Source: CAD feature listing. Evaluate the final solid. Frame: model axes, mm. A direction names the side the tool comes from. Give positions to 0.01 mm unless a question says otherwise; leave off trailing zeros. Loops run counter-clockwise (first coordinate to the right, second up) from the corner with the lowest first, then second, coordinate; pieces in that order, holes last. Notation, with made-up numbers: M -37.5,-9.5 L -31.5,-9.5 A15 cw -31.5,18.5 Z; hole C -26.75,33.25 d9. An arc over 180 degrees is marked long. Put each result on its own line as item: value. Start each with the question number.
```python
from build123d import *

# Parameters (mm, degrees)
SKETCH1_R           = 33.02
SKETCH1_R_2         = 22.225
BOSS_EXTRUDE1_DEPTH = 25.4
CAVITY1_DEPTH       = 25.4
CAVITY1_START       = 11.43
CAVITY1_2_DEPTH     = 2.54


# Read off the part's stored shape, not the designer's step: Cavity1
with BuildPart() as part:
    # Sketch1 → Boss-Extrude1 (new body)
    with BuildSketch(Plane(origin=(0, 0, 0), x_dir=(1, 0, 0), z_dir=(0, 1, 0))):
        with Locations(Location((0, 0, 0), (0, 0, 270))):
            Circle(SKETCH1_R)
        with Locations(Location((0, 0, 0), (0, 0, 270))):
            Circle(SKETCH1_R_2, mode=Mode.SUBTRACT)
    extrude(amount=BOSS_EXTRUDE1_DEPTH)

    # Cavity1 outline → Cavity1 (cut)
    with BuildSketch(Plane(origin=(0, 0, 0), x_dir=(1, 0, 0), z_dir=(0, 1, 0))):
        with BuildLine():
            Line((-6.35, -27.94), (6.35, -27.94))
            Line((6.35, -27.94), (2.54, -22.079380086))
            ThreePointArc((2.54, -22.079380086), (0, -22.225), (-2.54, -22.079380086))
            Line((-2.54, -22.079380086), (-6.35, -27.94))
        make_face()
        with BuildLine():
            Line((10.923030829, -19.355568256), (11.285462035, -26.336371175))
            Line((11.285462035, -26.336371175), (21.559977863, -18.871498471))
            Line((21.559977863, -18.871498471), (15.03283716, -16.369619174))
            ThreePointArc((15.03283716, -16.369619174), (13.063527232, -17.9804027), (10.923030829, -19.355568256))
        make_face()
        with BuildLine():
            Line((-11.285462035, -26.336371175), (-10.923030829, -19.355568256))
            ThreePointArc((-10.923030829, -19.355568256), (-13.063527232, -17.9804027), (-15.03283716, -16.369619174))
            Line((-15.03283716, -16.369619174), (-21.559977863, -18.871498471))
            Line((-21.559977863, -18.871498471), (-11.285462035, -26.336371175))
        make_face()
        with BuildLine():
            ThreePointArc((21.783641473, -4.407220121), (21.137231075, -6.8679027), (20.213835141, -9.238587223))
            Line((20.213835141, -9.238587223), (24.610261151, -14.673143701))
            Line((24.610261151, -14.673143701), (28.53477698, -2.594725944))
            Line((28.53477698, -2.594725944), (21.783641473, -4.407220121))
        make_face()
        with BuildLine():
            Line((-24.610261151, -14.673143701), (-20.213835141, -9.238587223))
            ThreePointArc((-20.213835141, -9.238587223), (-21.137231075, -6.8679027), (-21.783641473, -4.407220121))
            Line((-21.783641473, -4.407220121), (-28.53477698, -2.594725944))
            Line((-28.53477698, -2.594725944), (-24.610261151, -14.673143701))
        make_face()
        with BuildLine():
            Line((-28.53477698, 2.594725944), (-21.783641473, 4.407220121))
            ThreePointArc((-21.783641473, 4.407220121), (-21.137231075, 6.8679027), (-20.213835141, 9.238587223))
            Line((-20.213835141, 9.238587223), (-24.610261151, 14.673143701))
            Line((-24.610261151, 14.673143701), (-28.53477698, 2.594725944))
        make_face()
        with BuildLine():
            Line((21.783641473, 4.407220121), (28.53477698, 2.594725944))
            Line((28.53477698, 2.594725944), (24.610261151, 14.673143701))
            Line((24.610261151, 14.673143701), (20.213835141, 9.238587223))
            ThreePointArc((20.213835141, 9.238587223), (21.137231075, 6.8679027), (21.783641473, 4.407220121))
        make_face()
        with BuildLine():
            Line((-21.559977863, 18.871498471), (-15.03283716, 16.369619174))
            ThreePointArc((-15.03283716, 16.369619174), (-13.063527232, 17.9804027), (-10.923030829, 19.355568256))
            Line((-10.923030829, 19.355568256), (-11.285462035, 26.336371175))
            Line((-11.285462035, 26.336371175), (-21.559977863, 18.871498471))
        make_face()
        with BuildLine():
            ThreePointArc((10.923030829, 19.355568256), (13.063527232, 17.9804027), (15.03283716, 16.369619174))
            Line((15.03283716, 16.369619174), (21.559977863, 18.871498471))
            Line((21.559977863, 18.871498471), (11.285462035, 26.336371175))
            Line((11.285462035, 26.336371175), (10.923030829, 19.355568256))
        make_face()
        with BuildLine():
            Line((-6.35, 27.94), (-2.54, 22.079380086))
            ThreePointArc((-2.54, 22.079380086), (0, 22.225), (2.54, 22.079380086))
            Line((2.54, 22.079380086), (6.35, 27.94))
            Line((6.35, 27.94), (-6.35, 27.94))
        make_face()
    extrude(amount=CAVITY1_DEPTH, mode=Mode.SUBTRACT)

    # Cavity1 2 outline → Cavity1 2 (cut)
    with BuildSketch(Plane(origin=(0, 0, 0), x_dir=(1, 0, 0), z_dir=(0, 1, 0)).offset(CAVITY1_START)):
        with BuildLine():
            Line((2.54, -22.079380086), (5.935416317, -27.3022789))
            ThreePointArc((5.935416317, -27.3022789), (8.633934823, -26.572519065), (11.246024223, -25.576757793))
            Line((11.246024223, -25.576757793), (10.923030829, -19.355568256))
            ThreePointArc((10.923030829, -19.355568256), (6.8679027, -21.137231075), (2.54, -22.079380086))
        make_face()
        with BuildLine():
            ThreePointArc((-11.246024223, -25.576757793), (-8.633934823, -26.572519065), (-5.935416317, -27.3022789))
            Line((-5.935416317, -27.3022789), (-2.54, -22.079380086))
            ThreePointArc((-2.54, -22.079380086), (-6.8679027, -21.137231075), (-10.923030829, -19.355568256))
            Line((-10.923030829, -19.355568256), (-11.246024223, -25.576757793))
        make_face()
        with BuildLine():
            ThreePointArc((20.213835141, -9.238587223), (17.9804027, -13.063527232), (15.03283716, -16.369619174))
            Line((15.03283716, -16.369619174), (20.84972956, -18.599257438))
            ThreePointArc((20.84972956, -18.599257438), (22.603934823, -16.422719949), (24.131865747, -14.08178453))
            Line((24.131865747, -14.08178453), (20.213835141, -9.238587223))
        make_face()
        with BuildLine():
            Line((-20.84972956, -18.599257438), (-15.03283716, -16.369619174))
            ThreePointArc((-15.03283716, -16.369619174), (-17.9804027, -13.063527232), (-20.213835141, -9.238587223))
            Line((-20.213835141, -9.238587223), (-24.131865747, -14.08178453))
            ThreePointArc((-24.131865747, -14.08178453), (-22.603934823, -16.422719949), (-20.84972956, -18.599257438))
        make_face()
        with BuildLine():
            ThreePointArc((21.783641473, 4.407220121), (22.225, 0), (21.783641473, -4.407220121))
            Line((21.783641473, -4.407220121), (27.800154768, -2.7919518))
            ThreePointArc((27.800154768, -2.7919518), (27.94, 0), (27.800154768, 2.7919518))
            Line((27.800154768, 2.7919518), (21.783641473, 4.407220121))
        make_face()
        with BuildLine():
            Line((-27.800154768, -2.7919518), (-21.783641473, -4.407220121))
            ThreePointArc((-21.783641473, -4.407220121), (-22.225, 0), (-21.783641473, 4.407220121))
            Line((-21.783641473, 4.407220121), (-27.800154768, 2.7919518))
            ThreePointArc((-27.800154768, 2.7919518), (-27.94, 0), (-27.800154768, -2.7919518))
        make_face()
        with BuildLine():
            Line((-24.131865747, 14.08178453), (-20.213835141, 9.238587223))
            ThreePointArc((-20.213835141, 9.238587223), (-17.9804027, 13.063527232), (-15.03283716, 16.369619174))
            Line((-15.03283716, 16.369619174), (-20.84972956, 18.599257438))
            ThreePointArc((-20.84972956, 18.599257438), (-22.603934823, 16.422719949), (-24.131865747, 14.08178453))
        make_face()
        with BuildLine():
            ThreePointArc((15.03283716, 16.369619174), (17.9804027, 13.063527232), (20.213835141, 9.238587223))
            Line((20.213835141, 9.238587223), (24.131865747, 14.08178453))
            ThreePointArc((24.131865747, 14.08178453), (22.603934823, 16.422719949), (20.84972956, 18.599257438))
            Line((20.84972956, 18.599257438), (15.03283716, 16.369619174))
        make_face()
        with BuildLine():
            Line((-11.246024223, 25.576757793), (-10.923030829, 19.355568256))
            ThreePointArc((-10.923030829, 19.355568256), (-6.8679027, 21.137231075), (-2.54, 22.079380086))
            Line((-2.54, 22.079380086), (-5.935416317, 27.3022789))
            ThreePointArc((-5.935416317, 27.3022789), (-8.633934823, 26.572519065), (-11.246024223, 25.576757793))
        make_face()
        with BuildLine():
            ThreePointArc((2.54, 22.079380086), (6.8679027, 21.137231075), (10.923030829, 19.355568256))
            Line((10.923030829, 19.355568256), (11.246024223, 25.576757793))
            ThreePointArc((11.246024223, 25.576757793), (8.633934823, 26.572519065), (5.935416317, 27.3022789))
            Line((5.935416317, 27.3022789), (2.54, 22.079380086))
        make_face()
    extrude(amount=CAVITY1_2_DEPTH, mode=Mode.SUBTRACT)


solid = part.part
```
1. Contact query for flat-ended pins moving along their axis: pin 1 (3 mm diameter, centred on x = 13.5, y = 3.5, fed in from +Z); pin 2 (12 mm diameter, centred on y = 8.5, z = -23.5, fed in from +X); pin 3 (4 mm diameter, centred on y = 21.5, z = 0.5, fed in from +X). Output: stop coordinate, or through.
2. Section D-D, the plane x = -8. Output: boundary loops of the cut face in (y, z), plus the area to 3 significant figures.
3. Section B-B, the plane x = 0. Output: boundary loops of the cut face in (y, z).
4. Ray query, line 1 (Y direction, x = 4.5, z = -25); line 2 (X direction, y = 24.75, z = 23); line 3 (Z direction, x = 5.5, y = 22.25). Return the intervals inside material, ascending.
5. Section A-A, the plane z = 0. Output: boundary loops of the cut face in (x, y) (3 decimals).
6. Section C-C, the plane x = -16. Output: boundary loops of the cut face in (y, z), plus the area to 3 significant figures.
7. Set-up query: faces 1 (the face through (16.495, 12.522, -22.552)), 2 (the face through (-20, 11.43, 15)). Return all of +Z, -Z, +X, -X, +Y, -Y with unobstructed straight access to the full face (end or side cutting, diameter ignored); none if empty.
Results found:
1. pin 1: z = 30.76
1. pin 2: x = 28
1. pin 3: x = 33.02
2. outline: M 0,-32.04 L 25.4,-32.04 L 25.4,-20.74 L 13.97,-20.74 L 13.97,-26.77 L 11.43,-26.77 L 11.43,-20.74 L 0,-20.74 Z; M 0,20.74 L 11.43,20.74 L 11.43,26.77 L 13.97,26.77 L 13.97,20.74 L 25.4,20.74 L 25.4,32.04 L 0,32.04 Z
2. area: 543 mm²
3. outline: M 0,-33.02 L 25.4,-33.02 L 25.4,-27.94 L 0,-27.94 Z; M 0,27.94 L 25.4,27.94 L 25.4,33.02 L 0,33.02 Z
4. line 1: 0 to 11.43, 13.97 to 25.4
4. line 2: -23.69 to -15.88, -11.11 to -3.14, 3.14 to 11.11, 15.88 to 23.69
4. line 3: -32.56 to -27.94, -26.63 to -21.53, 21.53 to 26.63, 27.94 to 32.56
5. outline: M -33.02,0 L -22.225,0 L -22.225,11.43 L -27.94,11.43 L -27.94,13.97 L -22.225,13.97 L -22.225,25.4 L -33.02,25.4 Z; M 22.225,0 L 33.02,0 L 33.02,25.4 L 22.225,25.4 L 22.225,13.97 L 27.94,13.97 L 27.94,11.43 L 22.225,11.43 Z
6. outline: M 0,-28.88 L 25.4,-28.88 L 25.4,-22.91 L 0,-22.91 Z; M 0,-16.74 L 11.43,-16.74 L 11.43,-15.43 L 0,-15.43 Z; M 0,15.43 L 11.43,15.43 L 11.43,16.74 L 0,16.74 Z; M 0,22.91 L 25.4,22.91 L 25.4,28.88 L 0,28.88 Z; M 13.97,-16.74 L 25.4,-16.74 L 25.4,-15.43 L 13.97,-15.43 Z; M 13.97,15.43 L 25.4,15.43 L 25.4,16.74 L 13.97,16.74 Z
6. area: 364 mm²
7. face 1: +Y, -Y
7. face 2: none
